Input: part model. Units: mm. Frame: model coordinates. Coordinates: 2 decimals unless noted, no trailing zeros. Write each loop counter-clockwise with the first axis right and the second up, starting at its lowest first coordinate (ties: lowest second). Pieces come first, ordered by that corner, then holes.
1) Section query C-C (z = 15.5). Output: boundary loops of the cut face in (x, y).
2) Section query A-A (x = 0). Output: boundary loops of the cut face in (y, z).
3) Line query: L1, parallel to Y at x = -1, z = 8.75; L2, parallel to Z at x = 23, y = -2.5. Output: solid intervals per line, ascending.
4) Pin query (flat end, axial travel): pin 1 Ø3 at (x, z) = (6.5, 15) entering from +Y; pin 2 Ø10 at (x, z) = (-15, 7) entering from +Y; pin 3 Ø10 at (x, z) = (-5.5, 6.5) entering from +Y. Return the tip coordinate at first contact, or that it passes through.
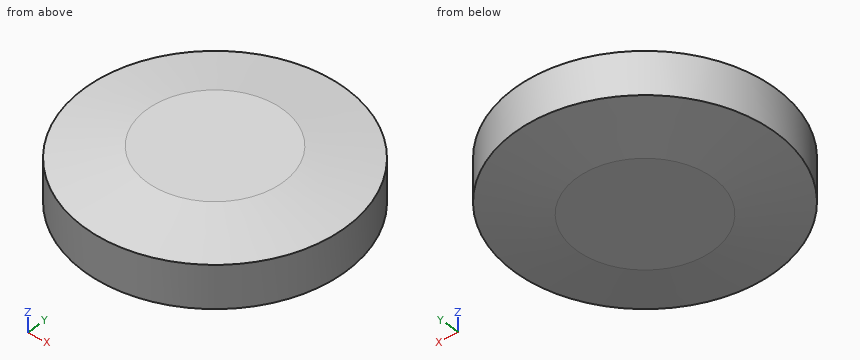
from build123d import *

# Parameters (mm, degrees)
F0_R       = 33.5
F1_DEPTH   = 17
F2_SIZE2   = 3
F2_SIZE    = 16
F2_2_SIZE2 = 3
F2_2_SIZE  = 16


with BuildPart() as f1:
    # F0 (on Top) → F1 (new body)
    with BuildSketch(Plane.XY):
        Circle(F0_R)
    extrude(amount=F1_DEPTH)

    # F2
    f2_edges = [f1.edges().sort_by_distance(p)[0] for p in [
        (-33.5, 0, 17),
    ]]
    f2_side = f1.faces().sort_by_distance((0, 0, 17))[0]
    chamfer(f2_edges, length=F2_SIZE, length2=F2_SIZE2, reference=f2_side)

    # F2#2
    f2_2_edges = [f1.edges().sort_by_distance(p)[0] for p in [
        (-33.5, 0, 0),
    ]]
    f2_2_side = f1.faces().sort_by_distance((0, 0, 0))[0]
    chamfer(f2_2_edges, length=F2_2_SIZE, length2=F2_2_SIZE2, reference=f2_2_side)


solid = f1.part
Answer:
1. outline: circle Ø51 at (0, 0)
2. outline: (-33.5, 3) - (-17.5, 0) - (17.5, 0) - (33.5, 3) - (33.5, 14) - (17.5, 17) - (-17.5, 17) - (-33.5, 14) - close
3. L1: y = -33.49 to 33.49
3. L2: z = 1.06 to 15.94
4. pin 1: stops at y = 33.06
4. pin 2: stops at y = 31.97
4. pin 3: stops at y = 33.5
